Can you work these out from the model? Positions are in its coordinate system, mm. A direction names the side the tool comes from. Round coordinates to 2 decimals unless told otherwise and drop trailing zeros. Order: outer loops, then holes, each group sorted by start corner. A loop starts at its lowest first (then second) coordinate and runs counter-clockwise, first axis right, second up. Notation, with made-up numbers: M 28,57.25 L 32,57.25 A31 cw 32,83.25 Z; hole C 60.5,-11 d1. An arc over 180 degrees is marked long. One line per question, with ' | ' between items.
Autodesk Inventor part; units mm, degrees
ref_plane "YZ Plane" through (0, 0, 0) normal (1, 0, 0) x (0, 1, 0)
ref_plane "XZ Plane" through (0, 0, 0) normal (0, 1, 0) x (-1, 0, 0)
ref_plane "XY Plane" through (0, 0, 0) normal (0, 0, 1) x (1, 0, 0)
sketch "Эскиз1" plane through (0, 0, 0) normal (0, 0, 1) x (1, 0, 0)
  line L0 (0, 0) -> (-6, 0) construction
  line L1 (-6, 0) -> (-6, -27.9727) construction
  line L2 (-6, -27.9727) -> (0, -27.9727) construction
  line L3 (0, -27.9727) -> (0, 0) construction
  line L4 (6, -39.5474) -> (6, -29.5474)
  line L5 (6, -29.5474) -> (-6, -29.5474)
  line L6 (-6, -29.5474) -> (-6, -39.5474)
  circle A0 centre (0, 0) radius 4.45
  circle A1 centre (0, 0) radius 40
  line L7 (29.5474, -6) -> (39.5474, -6)
  line L8 (29.5474, 6) -> (29.5474, -6)
  line L9 (39.5474, 6) -> (29.5474, 6)
  line L10 (6, 29.5474) -> (6, 39.5474)
  line L11 (-6, 29.5474) -> (6, 29.5474)
  line L12 (-6, 39.5474) -> (-6, 29.5474)
  line L13 (-29.5474, 6) -> (-39.5474, 6)
  line L14 (-29.5474, -6) -> (-29.5474, 6)
  line L15 (-39.5474, -6) -> (-29.5474, -6)
  line L16 (38.7298, 10) -> (-38.7298, 10)
  circle A2 centre (0, 0) radius 17.5
  line L17 (0, -40) -> (0, -31)
  line L18 (0, -31) -> (-6, -31)
  line L19 (0, -31) -> (6, -31)
  line L20 (5.5, -29.5474) -> (5.5, -39.6201)
  line L21 (-5.5, -29.5474) -> (-5.5, -39.6201)
  point P0 (6, -34.4819)
  point P1 (6, -27.9727)
  point P2 (6, -39.5474)
  point P3 (6, -39.5474)
  point P4 (-14.3614, 10)
  point P5 (14.3614, 10)
  point P6 (5.5, -31)
  point P7 (-5.5, -31)
  dimension "d1" = 6
  dimension "d2" = 12
  dimension "d3" = 10
  dimension "d6" = 8.9
  dimension "d12" = 80
  dimension "d15" = 360
  dimension "d19" = 35
  dimension "d24" = 9
  dimension "d25" = 0.5
ref_plane "РабПлоскость2" through (0, 0, 0.2) normal (0, 0, 1) x (1, 0, 0)
extrude "Выдавливание4" add sketch "Эскиз1" along normal blind 3.5 contours A2 L16 picked at (-0.1788, 8.1392)
extrude "Выдавливание5" add sketch "Эскиз1" along normal blind 11 contours A1 L20 L19 L4 | L4 L5 L6 A1 L15 L14 L13 L16 A2 L9 L8 L7 | L19 L20 L5 L4 | L7 L8 L9 A1 | L19 L18 L21 L5 L20 | A1 L6 L18 L21 | L21 L18 L6 L5 | A1 L13 L14 L15
properties part number "circle"
(1) If we section it at A-A on y = 0: Please give me the cut outline in (x, z).
Final values:
outline: M -40,0 L -4.45,0 L -4.45,3.5 L -17.5,3.5 L -17.5,11 L -40,11 Z; M 4.45,0 L 40,0 L 40,11 L 17.5,11 L 17.5,3.5 L 4.45,3.5 Z
(2) On a 3-axis mill with a long thin cutter (end or side, diameter ignored), from which of +Z, -Z, +X, -X, +Y, -Y can I reach the whole of each face in a straight line? I mean faces 1 (the flat face through (-1, -9, 0)), 2 (the flat face through (0, -7, 3.5)), 3 (the flat face through (-5.5, -35, 5)). Say none if no direction works.
Final values:
face 1: -Z, +X, -X, +Y, -Y | face 2: +Z | face 3: +Z, -Z, -Y
(3) If we section it at B-B on x = 0: Please give me the cut outline in (y, z), plus the area to 3 significant figures.
Final values:
outline: M -31,0 L -4.45,0 L -4.45,3.5 L -17.5,3.5 L -17.5,11 L -31,11 Z; M 4.45,0 L 10,0 L 10,3.5 L 4.45,3.5 Z | area: 214 mm^2
(4) Thinking about a two-plate mould opening in Y: for faces 4 (the cylindrical face through (0.53, -17.49, 7.2)), 5 (the flat face through (5.5, -35, 5)), 6 (the cylindrical face through (33.5, -21.86, 5.42)), 7 (the cylindrical face through (-0.965, 4.344, 1.726)), which applies, released by +Y, released by -Y, zero draft, split by the parting line, or undercut?
Final values:
face 4: undercut | face 5: zero draft | face 6: split by the parting line | face 7: undercut
(5) If we section it at D-D on z = 2: Please give me the cut outline in (x, y), plus the area to 3 significant figures.
Final values:
outline: M -38.73,10 A40 ccw -5.5,-39.62 L -5.5,-31 L 5.5,-31 L 5.5,-39.62 A40 ccw 38.73,10 Z; hole C 0,0 d8.9 | area: 3,150 mm^2
(6) Please list where these lines run through material, in increasing order: probe 1 along Y at (x, z) = (0, 1.3); probe 2 along X at (y, z) = (0, 9.5); probe 3 along Y at (x, z) = (0, 9.25). Write a range as [from, to].
Final values:
probe 1: [-31, -4.45], [4.45, 10] | probe 2: [-40, -17.5], [17.5, 40] | probe 3: [-31, -17.5]
(7) Will these pins go through, and if not, where does the flat tip stop? pin 1 Ø6 at (y, z) = (-9, 4) entering from -X; pin 2 Ø3 at (x, z) = (20.5, 5) entering from -Y; pin 3 Ø2 at (x, z) = (2.5, 5) entering from +Y; pin 4 Ø7 at (x, y) = (0, 0) entering from -Z.
Final values:
pin 1: x = -39.55 | pin 2: y = -35.2 | pin 3: y = -17.15 | pin 4: through
(8) If we section it at C-C on y = -32: Please give me the cut outline in (x, z).
Final values:
outline: M -24,0 L -5.5,0 L -5.5,11 L -24,11 Z; M 5.5,0 L 24,0 L 24,11 L 5.5,11 Z
